from build123d import *

# Parameters (mm, degrees)
SKETCH3_W               = 48
SKETCH3_H               = 14
BOSS_EXTRUDE2_DEPTH     = 14
SKETCH4_W               = 46
SKETCH4_H               = 12
CUT_EXTRUDE1_DEPTH      = 13
FILLET1_R               = 0.5
CUT_EXTRUDE2_DEPTH      = 32.112698372
CUT_EXTRUDE2_DEPTH_BACK = 32.112698372
SKETCH6_W               = 37
SKETCH6_H               = 4.5
SKETCH14_W              = 4
SKETCH14_H              = 1
CUT_EXTRUDE8_DEPTH      = 1.25
SKETCH15_W              = 1
SKETCH15_H              = 4
CUT_EXTRUDE9_DEPTH      = 1.25
CUT_EXTRUDE10_DEPTH     = 29.178005607
SKETCH20_W              = 1.2
SKETCH20_H              = 11
BOSS_EXTRUDE3_DEPTH     = 3
FILLET2_R               = 0.5
FILLET2_OF_MIRROR4_R    = 0.5
SKETCH24_R              = 2.75
CUT_EXTRUDE14_DEPTH     = 1
SKETCH25_W              = 0.6
SKETCH25_H              = 12
BOSS_EXTRUDE4_DEPTH     = 2.3
SKETCH28_W              = 8.4
SKETCH28_H              = 9.4
CUT_EXTRUDE15_DEPTH     = 0.4
SKETCH30_W              = 0.7
SKETCH30_H              = 12
BOSS_EXTRUDE6_DEPTH     = 11.75
CUT_EXTRUDE22_REACH     = 52.488
SKETCH38_W              = 0.5
SKETCH38_H              = 3.3
SKETCH39_W              = 0.6
SKETCH39_H              = 1.25
BOSS_EXTRUDE7_DEPTH     = 8.7
FILLET5_R               = 5
MIRROR5_START           = 3.325
MIRROR5_OUTLINE_W       = 0.4
MIRROR5_OUTLINE_H       = 9.4
MIRROR5_DEPTH           = 8.4
MIRROR5_START_2         = 11.725
MIRROR5_2_OUTLINE_W     = 1
MIRROR5_2_OUTLINE_H     = 3.3
MIRROR5_2_OUTLINE_W_2   = 0.7
MIRROR5_2_DEPTH         = 0.5
SKETCH36_W              = 0.7
SKETCH36_H              = 12
CUT_EXTRUDE23_DEPTH     = 11.75
SKETCH40_W              = 1.8
SKETCH40_H              = 12
CUT_EXTRUDE24_DEPTH     = 11
BOSS_EXTRUDE8_START     = 4
BOSS_EXTRUDE8_DEPTH     = 4
BOSS_EXTRUDE9_DEPTH     = 4


# Read off the part's stored shape, not the designer's step: Mirror5
with BuildPart() as part:
    # Sketch3 → Boss-Extrude2 (new body)
    with BuildSketch(Plane.XY):
        Rectangle(SKETCH3_W, SKETCH3_H)
    extrude(amount=BOSS_EXTRUDE2_DEPTH)

    # Sketch4 → Cut-Extrude1 (cut)
    with BuildSketch(Plane.XY.offset(14)):
        Rectangle(SKETCH4_W, SKETCH4_H)
    extrude(amount=-CUT_EXTRUDE1_DEPTH, mode=Mode.SUBTRACT)

    # Fillet1
    fillet1_edges = [part.edges().sort_by_distance(p)[0] for p in [
        (-24, 0, 14),
        (0, -7, 14),
        (24, 0, 14),
        (0, -7, 0),
        (-24, 0, 0),
        (0, 7, 0),
        (24, 0, 0),
        (24, -7, 7),
        (-24, -7, 7),
        (-24, 7, 7),
        (24, 7, 7),
        (0, 7, 14),
    ]]
    fillet(fillet1_edges, radius=FILLET1_R)

    # Sketch6 → Cut-Extrude2 (cut, two sides: drawn at the far end of the back side and taken through both)
    with BuildSketch(Plane.XZ.offset(7).offset(-CUT_EXTRUDE2_DEPTH_BACK)):
        with Locations((-2.7, 6.95)):
            Rectangle(SKETCH6_W, SKETCH6_H)
    extrude(amount=CUT_EXTRUDE2_DEPTH + CUT_EXTRUDE2_DEPTH_BACK, mode=Mode.SUBTRACT)

    # Sketch14 → Cut-Extrude8 (cut)
    with BuildSketch(Plane.XY.offset(14)):
        with Locations((0, 6.5)):
            Rectangle(SKETCH14_W, SKETCH14_H)
    cut_extrude8 = extrude(amount=-CUT_EXTRUDE8_DEPTH, mode=Mode.SUBTRACT)

    # Mirror1: Cut-Extrude8 across plane
    add(cut_extrude8.mirror(Plane(origin=(0, 0, 0), x_dir=(0, 0, 1), z_dir=(0, -1, 0))), mode=Mode.SUBTRACT)

    # Sketch15 → Cut-Extrude9 (cut)
    with BuildSketch(Plane.XY.offset(14)):
        with Locations((23.5, 0)):
            Rectangle(SKETCH15_W, SKETCH15_H)
    cut_extrude9 = extrude(amount=-CUT_EXTRUDE9_DEPTH, mode=Mode.SUBTRACT)

    # Mirror3: Cut-Extrude9 across plane
    add(cut_extrude9.mirror(Plane.ZY), mode=Mode.SUBTRACT)

    # Sketch17 → Cut-Extrude10 (cut, through all)
    with BuildSketch(Plane.XY.offset(1)):
        with BuildLine():
            Line((20, 4.675), (19.45, 4.675))
            ThreePointArc((19.45, 4.675), (18.389339828, 4.235660172), (17.95, 3.175))
            Line((17.95, 3.175), (17.95, -3.175))
            ThreePointArc((17.95, -3.175), (18.389339828, -4.235660172), (19.45, -4.675))
            Line((19.45, -4.675), (20, -4.675))
            ThreePointArc((20, -4.675), (21.060660172, -4.235660172), (21.5, -3.175))
            Line((21.5, -3.175), (21.5, 3.175))
            ThreePointArc((21.5, 3.175), (21.060660172, 4.235660172), (20, 4.675))
        make_face()
    extrude(amount=-CUT_EXTRUDE10_DEPTH, mode=Mode.SUBTRACT)

    # Sketch20 → Boss-Extrude3 (add)
    with BuildSketch(Plane(origin=(0, -6, 0), x_dir=(1, 0, 0), z_dir=(0, 1, 0))):
        with Locations((-21.8, -6.5)):
            Rectangle(SKETCH20_W, SKETCH20_H)
    boss_extrude3 = extrude(amount=BOSS_EXTRUDE3_DEPTH)

    # Fillet2
    fillet2_edges = [part.edges().sort_by_distance(p)[0] for p in [
        (-21.2, -3, 6.5),
        (-22.4, -3, 6.5),
    ]]
    fillet(fillet2_edges, radius=FILLET2_R)

    # Mirror4: Boss-Extrude3 across plane
    add(boss_extrude3.mirror(Plane(origin=(0, 0, 0), x_dir=(0, 0, 1), z_dir=(0, -1, 0))))

    # Fillet2 of Mirror4
    fillet2_of_mirror4_edges = [part.edges().sort_by_distance(p)[0] for p in [
        (-21.2, 3, 6.5),
        (-22.4, 3, 6.5),
    ]]
    fillet(fillet2_of_mirror4_edges, radius=FILLET2_OF_MIRROR4_R)

    # Sketch24 → Cut-Extrude14 (cut)
    with BuildSketch(Plane.ZY.offset(24)):
        with Locations((7, 0)):
            Circle(SKETCH24_R)
    extrude(amount=-CUT_EXTRUDE14_DEPTH, mode=Mode.SUBTRACT)

    # Sketch25 → Boss-Extrude4 (add)
    with BuildSketch(Plane.XY.offset(1)):
        with Locations((-22.7, 0)):
            Rectangle(SKETCH25_W, SKETCH25_H)
    extrude(amount=BOSS_EXTRUDE4_DEPTH)

    # Sketch28 → Cut-Extrude15 (cut)
    with BuildSketch(Plane(origin=(24, 0, 0), x_dir=(0, 0, -1), z_dir=(1, 0, 0))):
        with Locations((-7.525, 0)):
            Rectangle(SKETCH28_W, SKETCH28_H)
    extrude(amount=-CUT_EXTRUDE15_DEPTH, mode=Mode.SUBTRACT)

    # Sketch30 → Boss-Extrude6 (add)
    with BuildSketch(Plane.XY.offset(1)):
        with Locations((22.65, 0)):
            Rectangle(SKETCH30_W, SKETCH30_H)
    extrude(amount=BOSS_EXTRUDE6_DEPTH)

    # Cut-Extrude22: up to this face of the body (flat: up to its plane)
    cut_extrude22_end = Plane(part.part.faces().sort_by_distance((23, 4, 13.375))[0])
    # Sketch38 → Cut-Extrude22 (cut, up to the picked face)
    with BuildSketch(Plane(origin=(24, 0, 0), x_dir=(0, 0, -1), z_dir=(1, 0, 0)), mode=Mode.PRIVATE) as cut_extrude22_sk1:
        with Locations((-11.975, 0)):
            Rectangle(SKETCH38_W, SKETCH38_H)
    cut_extrude22_tool1 = split(extrude(cut_extrude22_sk1.sketch, amount=-CUT_EXTRUDE22_REACH, mode=Mode.PRIVATE), bisect_by=cut_extrude22_end, keep=Keep.BOTH, mode=Mode.PRIVATE)
    add(cut_extrude22_tool1.solids().sort_by(Axis((24, 0, 11.975), (-1, 0, 0)))[0], mode=Mode.SUBTRACT)

    # Sketch39 → Boss-Extrude7 (add)
    with BuildSketch(Plane.XY.offset(3.3)):
        with Locations((-22.7, 5.375)):
            Rectangle(SKETCH39_W, SKETCH39_H)
        with Locations((-22.7, -5.375)):
            Rectangle(SKETCH39_W, SKETCH39_H)
    extrude(amount=BOSS_EXTRUDE7_DEPTH)

    # Fillet5
    # the kernel refuses this fillet: 5 mm, written as the material it takes off along each edge
    with BuildSketch(Plane(origin=(-23, 4.75, 12), x_dir=(0, 1, 0), z_dir=(1, 0, 0))) as fillet5_piece_1:
        with BuildLine():
            CenterArc((5, -3.307189139), FILLET5_R, 138.590377891, 41.409622109)
            Line((0, -3.307189139), (0, 0))
            Line((0, 0), (1.25, 0))
        make_face()
    extrude(amount=0.6, mode=Mode.SUBTRACT)
    with BuildSketch(Plane(origin=(-23, -4.75, 12), x_dir=(0, 0, -1), z_dir=(1, 0, 0))) as fillet5_piece_2:
        with BuildLine():
            CenterArc((3.307189139, -5), FILLET5_R, 90, 41.409622109)
            Line((0, -1.25), (0, 0))
            Line((0, 0), (3.307189139, 0))
        make_face()
    extrude(amount=0.6, mode=Mode.SUBTRACT)

    # Mirror5 outline → Mirror5 (cut)
    with BuildSketch(Plane.XY.offset(MIRROR5_START)):
        with Locations((-23.8, 0)):
            Rectangle(MIRROR5_OUTLINE_W, MIRROR5_OUTLINE_H)
    extrude(amount=MIRROR5_DEPTH, mode=Mode.SUBTRACT)

    # Mirror5 2 outline → Mirror5 2 (cut)
    with BuildSketch(Plane.XY.offset(MIRROR5_START_2)):
        with Locations((-23.5, 0)):
            Rectangle(MIRROR5_2_OUTLINE_W, MIRROR5_2_OUTLINE_H)
        with Locations((22.65, 0)):
            Rectangle(MIRROR5_2_OUTLINE_W_2, MIRROR5_2_OUTLINE_H)
    extrude(amount=MIRROR5_2_DEPTH, mode=Mode.SUBTRACT)

    # Sketch36 → Cut-Extrude23 (cut)
    with BuildSketch(Plane.XY.offset(12.75)):
        with Locations((22.65, 0)):
            Rectangle(SKETCH36_W, SKETCH36_H)
    extrude(amount=-CUT_EXTRUDE23_DEPTH, mode=Mode.SUBTRACT)

    # Sketch40 → Cut-Extrude24 (cut)
    with BuildSketch(Plane.XY.offset(12)):
        with Locations((-22.1, 0)):
            Rectangle(SKETCH40_W, SKETCH40_H)
    extrude(amount=-CUT_EXTRUDE24_DEPTH, mode=Mode.SUBTRACT)

    # Sketch41 → Boss-Extrude8 (add)
    with BuildSketch(Plane(origin=(0, -2, 0), x_dir=(1, 0, 0), z_dir=(0, 1, 0)).offset(BOSS_EXTRUDE8_START)):
        with BuildLine():
            Line((24, -13.5), (23, -13.5))
            Line((23, -13.5), (23, -14))
            Line((23, -14), (23.5, -14))
            ThreePointArc((23.5, -14), (23.853553391, -13.853553391), (24, -13.5))
        make_face()
    boss_extrude8 = extrude(amount=-BOSS_EXTRUDE8_DEPTH)

    # Mirror6: Boss-Extrude8 across plane
    add(boss_extrude8.mirror(Plane.ZY))

    # Sketch42 → Boss-Extrude9 (add)
    with BuildSketch(Plane.ZY.offset(-2)):
        with BuildLine():
            Line((14, -6), (14, -6.5))
            ThreePointArc((14, -6.5), (13.853553391, -6.853553391), (13.5, -7))
            Line((13.5, -7), (13.5, -6))
            Line((13.5, -6), (14, -6))
        make_face()
    boss_extrude9 = extrude(amount=BOSS_EXTRUDE9_DEPTH)

    # Mirror7: Boss-Extrude9 across plane
    add(boss_extrude9.mirror(Plane(origin=(0, 0, 0), x_dir=(0, 0, 1), z_dir=(0, -1, 0))))


solid = part.part
For this review, take the finished solid that the model builds, in its own axes (mm). A direction names the side the tool comes from. Coordinates: 2 decimals unless noted, no trailing zeros. Write each loop counter-clockwise with the first axis right and the second up, starting at its lowest first coordinate (ties: lowest second). Pieces come first, ordered by that corner, then holes. Notation, with made-up numbers: (44, 25.25) -> (72, 25.25) arc R30 ccw to (72, 63.25) -> close; hole circle Ø7 at (-19.75, 74.5). An arc over 180 degrees is marked (long way). Write each question's results on one line, items separated by ' | '. Start each with the question number.
1) Insertion check: pin 1 (1.5 mm diameter, centred on x = -17, y = 2.5, fed in from +Z); pin 2 (6 mm diameter, centred on y = -0.5, z = 7.5, fed in from -X); pin 3 (7 mm diameter, centred on y = 0, z = 7, fed in from +X). Each pin has a flat end and moves straight along its axis. Give the tip position at first contact, or say it passes through.
2) Consider section B-B (x = -18). Write out the cut boundary in (y, z).
3) Wall thickness on L1, parallel to Y at x = -1.5, z = 11.25; L2, parallel to X at y = 5.25, z = 12.75; L3, parallel to X at y = 2.5, z = 11: over which ranges is each line inside the solid? List them lowest first. Write a range as [from, to].
4) Consider section D-D (y = -4). Write out the cut boundary in (x, z) (3 decimals), plus the area to 3 significant figures.
5) Consider section A-A (z = 7). Give the number of separate pieces and of enclosed holes in the cut face, plus the area to 3 significant figures.
6) The part is to be moulded in two halves that separate along X. For faces 1 (the face through (-23.6, 0, 10)), 2 (the face through (0.3, 6, 4.5)), 3 (the face through (23.5, 0, 12.225)), say which applies: +X half, -X half, draft (parallel to the pull), parting line (faces both ways), or undercut.
7) For faces 4 (the face through (0, 6.5, 12.75)), 5 (the face through (-23.5, 0, 12.75)), 6 (the face through (-23.3, -1.05, 9.54)), list the 3-axis set-ups (+Z, -Z, +X, -X, +Y, -Y) from which the entire face can be reached by the end or side of a thin tool; tool diameter is ignored.
Geometry says:
1) pin 1: z = 1 | pin 2: x = -23.6 | pin 3: x = 23.6
2) outline: (-7, 0.5) arc R0.5 ccw to (-6.5, 0) -> (6.5, 0) arc R0.5 ccw to (7, 0.5) -> (7, 4.7) -> (6, 4.7) -> (6, 1) -> (-6, 1) -> (-6, 4.7) -> (-7, 4.7) -> close; (-7, 9.2) -> (-6, 9.2) -> (-6, 14) -> (-6.5, 14) arc R0.5 ccw to (-7, 13.5) -> close; (6, 9.2) -> (7, 9.2) -> (7, 13.5) arc R0.5 ccw to (6.5, 14) -> (6, 14) -> close
3) L1: [-7, -6], [6, 7] | L2: [-24, -23], [23, 24] | L3: [-23.6, -23], [23, 23.6]
4) outline: (-24, 0.5) arc R0.5 ccw to (-23.5, 0) -> (18.197, 0) -> (18.197, 1) -> (-23, 1) -> (-23, 14) -> (-23.5, 14) arc R0.5 ccw to (-24, 13.5) -> (-24, 11.725) -> (-23.6, 11.725) -> (-23.6, 3.325) -> (-24, 3.325) -> close; (21.253, 0) -> (23.5, 0) arc R0.5 ccw to (24, 0.5) -> (24, 3.325) -> (23.6, 3.325) -> (23.6, 11.725) -> (24, 11.725) -> (24, 13.5) arc R0.5 ccw to (23.5, 14) -> (23, 14) -> (23, 1) -> (21.253, 1) -> close | area: 64.0 mm^2
5) separate pieces: 3 | enclosed holes: 0 | area: 35.0 mm^2
6) face 1: -X half | face 2: undercut | face 3: draft
7) face 4: +Y, -Y | face 5: +X, -X | face 6: -X
